from build123d import *

# Parameters (mm, degrees)
SKETCH_1_R          = 2.55
SKETCH_1_R_2        = 7.5
EXTRUDE_1_DEPTH     = 5
FILLET_1_R          = 20
FILLET_2_R          = 5
CUT_EXTRUDE_1_DEPTH = 109.559891304
EXTRUDE_2_DEPTH     = 5
SKETCH_3_R          = 1.55
CUT_EXTRUDE_2_DEPTH = 109.559891304
FILLET_3_R          = 2
SKETCH_5_R          = 3
CUT_EXTRUDE_3_DEPTH = 3


with BuildPart() as part:
    # ｽｹｯﾁ1 → ﾎﾞｽ - 押し出し1 (new body)
    with BuildSketch(Plane(origin=(0, 0, 0), x_dir=(1, 0, 0), z_dir=(0, 1, 0))):
        with BuildLine():
            Line((0, 0), (0, -48))
            ThreePointArc((0, -48), (12.5, -60.5), (25, -48))
            Line((25, -48), (25, -20))
            Line((25, -20), (90, -20))
            Line((90, -20), (90, 30))
            Line((90, 30), (0, 0))
        make_face()
        with Locations(Location((75.769750529, 14.715657976, 0), (0, 0, 270))):
            Circle(SKETCH_1_R, mode=Mode.SUBTRACT)
        with Locations(Location((75, -10, 0), (0, 0, 270))):
            Circle(SKETCH_1_R, mode=Mode.SUBTRACT)
        with Locations(Location((25, -10, 0), (0, 0, 270))):
            Circle(SKETCH_1_R, mode=Mode.SUBTRACT)
        with Locations(Location((12.5, -48, 0), (0, 0, 270))):
            Circle(SKETCH_1_R_2, mode=Mode.SUBTRACT)
    extrude(amount=EXTRUDE_1_DEPTH)

    # ﾌｨﾚｯﾄ1
    fillet_1_edges = [part.edges().sort_by_distance(p)[0] for p in [
        (25, 2.5, 20),
    ]]
    fillet(fillet_1_edges, radius=FILLET_1_R)

    # ﾌｨﾚｯﾄ2
    fillet_2_edges = [part.edges().sort_by_distance(p)[0] for p in [
        (90, 2.5, -30),
        (90, 2.5, 20),
    ]]
    fillet(fillet_2_edges, radius=FILLET_2_R)

    # ｽｹｯﾁ2 → ｶｯﾄ - 押し出し1 (cut, through all)
    with BuildSketch(Plane(origin=(0, 5, 0), x_dir=(1, 0, 0), z_dir=(0, 1, 0))):
        with BuildLine():
            Line((3.3, -48), (3.3, -34))
            ThreePointArc((3.3, -34), (3.592893219, -33.292893219), (4.3, -33))
            Line((4.3, -33), (20.7, -33))
            ThreePointArc((20.7, -33), (21.407106781, -33.292893219), (21.7, -34))
            Line((21.7, -34), (21.7, -48))
            ThreePointArc((21.7, -48), (12.5, -57.2), (3.3, -48))
        make_face()
    extrude(amount=-CUT_EXTRUDE_1_DEPTH, mode=Mode.SUBTRACT)

    # ｽｹｯﾁ4 → ﾎﾞｽ - 押し出し2 (add)
    with BuildSketch(Plane(origin=(0, 5, 0), x_dir=(1, 0, 0), z_dir=(0, 1, 0))):
        Polygon((0, 0), (0, 20), (60, 20), align=None)
    extrude(amount=-EXTRUDE_2_DEPTH)

    # ｽｹｯﾁ3 → ｶｯﾄ - 押し出し2 (cut, through all)
    with BuildSketch(Plane(origin=(0, 5, 0), x_dir=(1, 0, 0), z_dir=(0, 1, 0))):
        with Locations(Location((20.5, 5, 0), (0, 0, 270))):
            Circle(SKETCH_3_R)
        with Locations(Location((4.5, 5, 0), (0, 0, 90))):
            Circle(SKETCH_3_R)
    extrude(amount=-CUT_EXTRUDE_2_DEPTH, mode=Mode.SUBTRACT)

    # ﾌｨﾚｯﾄ3
    fillet_3_edges = [part.edges().sort_by_distance(p)[0] for p in [
        (60, 2.5, -20),
        (0, 2.5, -20),
    ]]
    fillet(fillet_3_edges, radius=FILLET_3_R)

    # ｽｹｯﾁ5 → ｶｯﾄ - 押し出し3 (cut)
    with BuildSketch(Plane.XZ.offset(-5)):
        with Locations(Location((4.5, -5, 0), (0, 0, 270))):
            Circle(SKETCH_5_R)
        with Locations(Location((20.5, -5, 0), (0, 0, 270))):
            Circle(SKETCH_5_R)
    extrude(amount=CUT_EXTRUDE_3_DEPTH, mode=Mode.SUBTRACT)


solid = part.part
CAD build for the part. Positions are in the model's coordinates, mm. A direction names the side the tool comes from. Round coordinates to 2 decimals unless told otherwise and drop trailing zeros. Loops run counter-clockwise (first coordinate to the right, second up) from the corner with the lowest first, then second, coordinate; pieces in that order, holes last.
(1) Cut at A-A (x = 12.5). Give the cut face in (y, z).
(2) Cut at D-D (x = 57). Give the cut face in (y, z).
(3) Cut at B-B (z = 10). Give the cut face in (x, y).
(4) Which spindle directions (+Z, -Z, +X, -X, +Y, -Y) get a long thin tool onto all of the face, cutting with end or side? Do faces 5 (the flat face through (19, 2, -6)), 6 (the flat face through (3.3, 3, 41)), 7 (the flat face through (25, 2, 44)), 8 (the cylindrical face through (0.57, 2.46, -19.4)). Say none if no direction does.
(5) Two-plate mould, pull along Z, no slides. Class faces 1 (the flat face through (12, 3, 33)), 2 (the flat face through (65, 2, 20)), 3 (the flat face through (46, 0, 6)), 4 (the flat face through (21.7, 3, 41)): +Z half, -Z half, draft (parallel to the pull), parting line (faces both ways), or undercut.
(6) Cut at C-C (y = 3.6). Give the cut face in (x, z).
(7) Wall check: line 1 along X through (y, z) = (4.45, -5); line 2 along X through (y, z) = (0.7, -5); line 3 along Z through (x, y) = (4.5, 1.3). Give the ranges that are in metal, low to high.
(8) Drop flat-ended pins along their axis: pin 1 (1.5 mm diameter, centred on x = 23, y = 2, fed in from -Z); pin 2 (1.5 mm diameter, centred on x = 58, y = 1.5, fed in from +Z); pin 3 (1.5 mm diameter, centred on y = 3, z = 39.5, fed in from +X). Give the stop position or say it passes through.
Findings below:
1. outline: (0, -20) - (5, -20) - (5, 33) - (0, 33) - close; (0, 57.2) - (5, 57.2) - (5, 60.5) - (0, 60.5) - close
2. outline: (0, -20) - (5, -20) - (5, 20) - (0, 20) - close
3. outline: (0, 0) - (22.45, 0) - (22.45, 5) - (0, 5) - close; (27.55, 0) - (72.45, 0) - (72.45, 5) - (27.55, 5) - close; (77.55, 0) - (90, 0) - (90, 5) - (77.55, 5) - close
4. face 5: +Y
4. face 6: +Y, -Y
4. face 7: +Z, +X, +Y, -Y
4. face 8: -Z, -X, +Y, -Y
5. face 1: undercut
5. face 2: +Z half
5. face 3: draft
5. face 4: undercut
6. outline: (0, -18) arc R2 ccw to (2, -20) - (59.68, -20) arc R2 cw to (60.31, -20.1) - (83.42, -27.81) arc R5 ccw to (90, -23.06) - (90, 15) arc R5 ccw to (85, 20) - (45, 20) arc R20 cw to (25, 40) - (25, 48) arc R12.5 ccw to (0, 48) - close; hole circle Ø6 at (4.5, -5); hole (3.3, 34) arc R1 ccw to (4.3, 33) - (20.7, 33) arc R1 ccw to (21.7, 34) - (21.7, 48) arc R9.2 ccw to (3.3, 48) - close; hole circle Ø6 at (20.5, -5); hole circle Ø5.1 at (25, 10); hole circle Ø5.1 at (75, 10); hole circle Ø5.1 at (75.77, -14.72)
7. line 1: x = 0 to 1.5, 7.5 to 17.5, 23.5 to 90
7. line 2: x = 0 to 2.95, 6.05 to 18.95, 22.05 to 90
7. line 3: z = -20 to -6.55, -3.45 to 33, 52.54 to 57.6
8. pin 1: stops at z = -20
8. pin 2: stops at z = 20
8. pin 3: stops at x = 25.04
